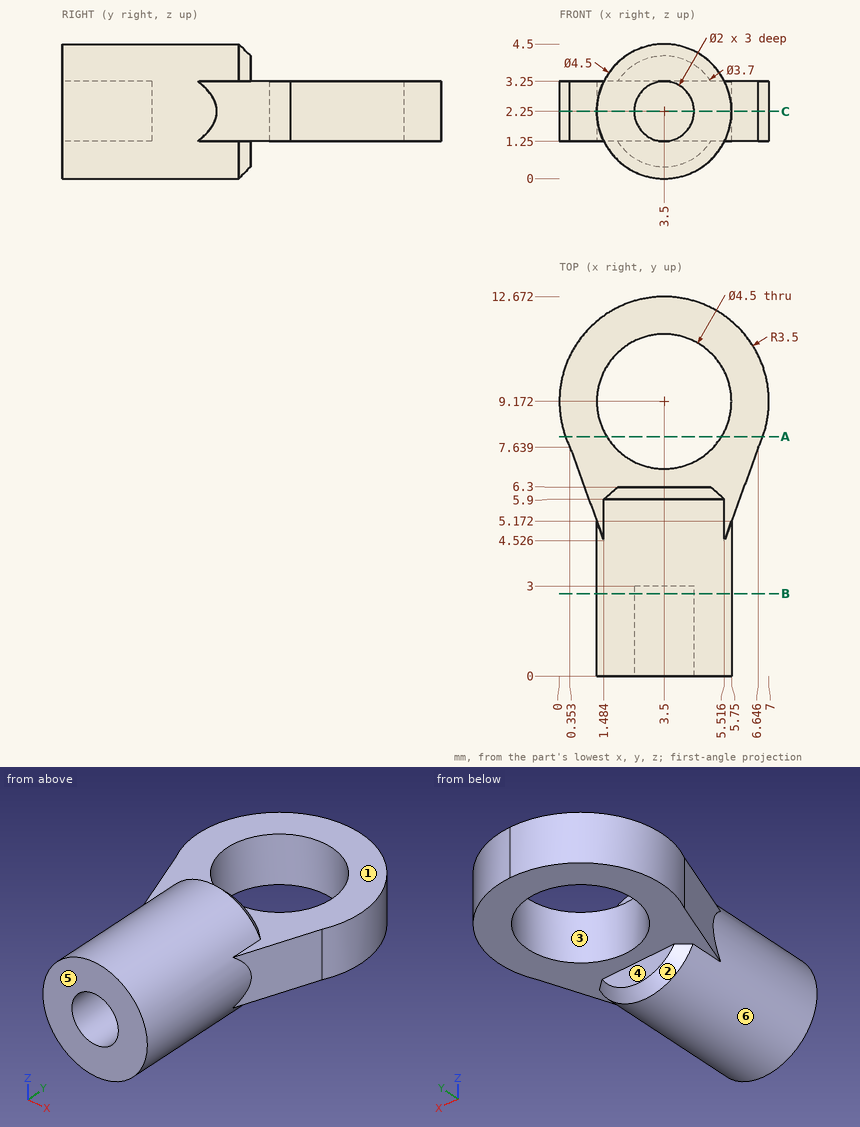
Here's the drawing with two shaded views (mm, measured from the low corner). I have some questions. A direction names the side the tool comes from. Give positions to 0.01 mm unless a question says otherwise; leave off trailing zeros. Loops run counter-clockwise (first coordinate to the right, second up) from the corner with the lowest first, then second, coordinate; pieces in that order, holes last. Notation, with made-up numbers: (-9, 81.5) -> (13, 81.5) arc R20 ccw to (13, 109.5) -> close; hole circle Ø1 at (19.5, 52.25). An arc over 180 degrees is marked (long way). One line per item, written item: value.
Q1. We'd pull the mould along Y, two halves only. Please class the marked faces 1, 2 and 3: pulls with the +Y half, pulls with the -Y half, needs draft (parallel to the pull), parting line crosses it, or undercut.
Answers follow:
face 1: needs draft
face 2: pulls with the +Y half
face 3: undercut
Q2. If I drill on line 1 along X through (y, z) = (4.5, 2.3); line 2 along Y through (x, z) = (3.5, 0.6); line 3 along Y through (x, z) = (4, 1.6) (1 decimal), over which ranges is the centre line in solid material (lowest first)?
Answers follow:
line 1: 1.25 to 5.75
line 2: 0 to 6.3
line 3: 3 to 7, 11.4 to 12.6
Q3. I'm going to push a flat-ended pin straight in: pin 1 Ø1.5 at (x, y) = (5, 6) entering from +Z. Where does the tip first touch, or does it pass through?
Answers follow:
pin 1: z = 4.37
Q4. Suppose I cut it at A-A on y = 8. Please give me the cut outline in (x, z).
Answers follow:
outline: (0.2, 1.25) -> (1.58, 1.25) -> (1.58, 3.25) -> (0.2, 3.25) -> close; (5.42, 1.25) -> (6.8, 1.25) -> (6.8, 3.25) -> (5.42, 3.25) -> close
Q5. On a 3-axis mill with a long thin cutter (end or side, diameter ignored), from which of +Z, -Z, +X, -X, +Y, -Y can I reach the whole of each face in a straight line? I mean the marked faces 4, 5 and 6. Say none if no direction works.
Answers follow:
face 4: -Z, +X, -X, +Y
face 5: +Z, -Z, +X, -X, -Y
face 6: -Y
Q6. Suppose I cut it at C-C on z = 2.25. Please give me the cut outline in (x, y).
Answers follow:
outline: (0.35, 7.64) -> (1.25, 5.17) -> (1.25, 0) -> (2.5, 0) -> (2.5, 3) -> (4.5, 3) -> (4.5, 0) -> (5.75, 0) -> (5.75, 5.17) -> (6.65, 7.64) arc R3.5 ccw to (3.5, 12.67) arc R3.5 ccw to start; hole circle Ø4.5 at (3.5, 9.17)
Q7. Suppose I cut it at B-B on y = 2.75. Please give me the cut outline in (x, z).
Answers follow:
outline: circle Ø4.5 at (3.5, 2.25); hole circle Ø2 at (3.5, 2.25)
